Geometry: final body of the model. Coordinates: model frame, mm. Face numbers are marked on the shaded views. A direction names the side the tool comes from. Give positions to 0.01 mm unless a question says otherwise; leave off trailing zeros. Write each loop counter-clockwise with the first axis right and the second up, starting at its lowest first coordinate (ties: lowest second). Pieces come first, ordered by that corner, then holes. Notation, with made-up numbers: M 41.5,56 L 49.5,56 A25 cw 49.5,69 Z; hole C 39.25,-1.75 d2. An arc over 180 degrees is marked long. Use a Markdown table: item, result. Add a question column.
(1) Reachability of the marked faces 3 and 4 from +Z, -Z, +X, -X, +Y, -Y: full face, straight path, thin tool, end or side. Return the list, or none.
(2) Cut plane C-C (x = -583.5). Output: boundary loops of the cut face in (y, z).
(3) Draft query along Z for the marked faces 1 and 2. Return one class per face: released by +Z, released by -Z, zero draft, split by the parting line, or undercut.
(4) Cut plane D-D (z = -69.5). Output: boundary loops of the cut face in (x, y).
(5) Material intervals for L1, parallel to X at y = 31, z = -332.5; L2, parallel to Z at x = -277.5, y = 37.5; L3, parallel to Z at x = -638, y = 11.5, sorted ascending.
(6) Pin query (flat end, axial travel): pin 1 Ø12 at (x, z) = (-270, -61.5) entering from +Y; pin 2 Ø3.5 at (y, z) = (54, -441.5) entering from -X; pin 3 Ø2 at (y, z) = (14.5, -516.5) entering from +X; pin 4 Ø3.5 at (x, y) = (-68.5, 58.5) entering from +Z. Return the tip coordinate at first contact, or that it passes through.
(7) Cut plane B-B (x = -392). Output: boundary loops of the cut face in (y, z), plus the area to 3 significant figures.
(8) Cut plane A-A (z = -234). Output: boundary loops of the cut face in (x, y), plus the area to 3 significant figures.
Autodesk Inventor part; units mm, degrees
ref_plane "YZ Plane" through (0, 0, 0) normal (1, 0, 0) x (0, 1, 0)
ref_plane "XZ Plane" through (0, 0, 0) normal (0, 1, 0) x (-1, 0, 0)
ref_plane "XY Plane" through (0, 0, 0) normal (0, 0, 1) x (1, 0, 0)
sketch "Skizze1" plane through (0, 0, 0) normal (0, 1, 0) x (-1, 0, 0)
  line L0 (0, 0) -> (80, 0)
  line L1 (80, 0) -> (80, -650)
  line L2 (80, -650) -> (0, -650)
  line L3 (0, -650) -> (0, 0)
  line L4 (80, -570) -> (80, -650)
  line L5 (80, -650) -> (570, -650)
  line L6 (570, -650) -> (570, -570)
  line L7 (570, -570) -> (80, -570)
  line L8 (80, -570) -> (80, -650)
  line L9 (80, 0) -> (570, 0)
  line L10 (570, 0) -> (570, -80)
  line L11 (570, -80) -> (80, -80)
  line L12 (80, -80) -> (80, 0)
  line L13 (570, 0) -> (650, 0)
  line L14 (650, 0) -> (650, -650)
  line L15 (650, -650) -> (570, -650)
  line L16 (570, -650) -> (570, 0)
  dimension "d0" = 80
  dimension "d1" = 650
  dimension "d4" = 490
  dimension "d5" = 80
  dimension "d6" = 80
  dimension "d7" = 80
extrude "Extrusion1" add sketch "Skizze1" along normal blind 80 contours L0 L1 L2 L3 | L9 L10 L11 L1 | L13 L14 L15 L6 L16 L10 | L1 L7 L6 L5
sketch "Skizze2" plane through (0, 80, 0) normal (0, 1, 0) x (1, 0, 0)
  line L0 (0, 0) -> (0, 650)
  line L1 (0, 650) -> (-650, 650)
  line L2 (-650, 650) -> (-650, 0)
  line L3 (-650, 0) -> (0, 0)
  line L4 (-80, 80) -> (-570, 80)
  line L5 (-570, 80) -> (-570, 570)
  line L6 (-570, 570) -> (-80, 570)
  line L7 (-80, 570) -> (-80, 80)
  line L8 (-490, 305) -> (-490, 345)
  line L9 (-490, 345) -> (-650, 345)
  line L10 (-650, 345) -> (-650, 305)
  line L11 (-650, 305) -> (-490, 305)
  line L12 (-570, 80) -> (-570, 570)
  line L13 (-490, 305) -> (-650, 345) construction
  line L14 (-490, 345) -> (-650, 305) construction
  line L15 (-80, 80) -> (-570, 80)
  line L16 (-570, 80) -> (-270, 80)
  line L17 (-250, 160) -> (-290, 160)
  line L18 (-290, 160) -> (-290, 0)
  line L19 (-290, 0) -> (-250, 0)
  line L20 (-250, 0) -> (-250, 160)
  line L21 (-250, 160) -> (-290, 0) construction
  line L22 (-290, 160) -> (-250, 0) construction
  line L23 (-650, 325) -> (0, 325)
  line L24 (-250, 490) -> (-290, 490)
  line L25 (-290, 490) -> (-290, 650)
  line L26 (-250, 650) -> (-250, 490)
  line L27 (-290, 650) -> (-250, 650)
  point P0 (-570, 325)
  point P1 (-250, 570)
  point P2 (-290, 570)
  point P3 (-570, 345)
  point P4 (-570, 305)
  point P5 (-250, 80)
  point P6 (-290, 80)
  dimension "d10" = 40
  dimension "d11" = 300
  dimension "d12" = 40
extrude "Extrusion2" cut sketch "Skizze2" against normal blind 30 contours L3 L18 L4 L20 | L26 L6 L25 L1 | L23 L2 L9 L5 | L5 L11 L2 L23
sketch "Skizze3" plane through (0, 50, 0) normal (0, 1, 0) x (1, 0, 0)
  line L0 (-290, 80) -> (-250, 80)
  line L1 (-290, 0) -> (-290, 80)
  line L2 (-250, 0) -> (-290, 0)
  line L3 (-250, 80) -> (-250, 0)
  line L4 (-290, 650) -> (-250, 650)
  line L5 (-290, 570) -> (-290, 650)
  line L6 (-250, 570) -> (-290, 570)
  line L7 (-250, 650) -> (-250, 570)
  line L8 (-650, 345) -> (-570, 345)
  line L9 (-650, 305) -> (-650, 345)
  line L10 (-570, 305) -> (-650, 305)
  line L11 (-570, 345) -> (-570, 305)
  line L12 (-650, 305) -> (-625, 305)
  line L13 (-570, 305) -> (-650, 305)
  line L14 (-625, 305) -> (-625, 345)
  line L15 (-290, 650) -> (-290, 625)
  line L16 (-290, 570) -> (-290, 650)
  line L17 (-290, 625) -> (-250, 625)
  line L18 (-290, 0) -> (-290, 25)
  line L19 (-290, 25) -> (-250, 25)
  point P0 (0, 0)
  dimension "d15" = 25
  dimension "d16" = 25
  dimension "d17" = 25
extrude "Extrusion3" cut sketch "Skizze3" against normal blind 5 contours L0 L3 L19 L1 | L17 L7 L6 L5 | L8 L11 L10 L14
sketch "Skizze4" plane through (0, 0, -650) normal (0, 0, -1) x (-1, 0, 0)
  line L0 (290, 80) -> (290, 50)
  line L1 (290, 50) -> (250, 50)
  line L2 (250, 50) -> (250, 80)
  line L3 (0, 80) -> (250, 80)
  line L4 (0, 0) -> (0, 80)
  line L5 (0, 0) -> (650, 0)
  line L6 (650, 0) -> (650, 80)
  line L7 (290, 80) -> (650, 80)
  line L8 (250, 50) -> (250, 45)
  line L9 (250, 50) -> (0, 50)
  line L10 (0, 0) -> (0, 80)
  line L11 (290, 50) -> (250, 50)
  line L12 (250, 50) -> (250, 62)
  line L13 (250, 62) -> (0, 62)
  line L14 (290, 50) -> (650, 50)
  line L15 (290, 62) -> (650, 62)
  dimension "d20" = 12
extrude "Extrusion4" cut sketch "Skizze4" against normal blind 12 contours L15 L6 L14 L0 | L9 L4 L13 L2
sketch "Skizze5" plane through (-650, 0, -650) normal (-1, 0, 0) x (0, 0, 1)
  line L0 (12, 50) -> (0, 50)
  line L1 (0, 0) -> (0, 50)
  line L2 (0, 0) -> (650, 0)
  line L3 (650, 0) -> (650, 80)
  line L4 (345, 80) -> (650, 80)
  line L5 (345, 80) -> (345, 50)
  line L6 (345, 50) -> (305, 50)
  line L7 (305, 50) -> (305, 80)
  line L8 (0, 80) -> (305, 80)
  line L9 (0, 62) -> (0, 80)
  line L10 (0, 62) -> (12, 62)
  line L11 (12, 62) -> (12, 50)
  line L12 (12, 50) -> (650, 50)
  line L13 (12, 62) -> (650, 62)
  point P0 (345, 62)
  point P1 (305, 62)
extrude "Extrusion5" cut sketch "Skizze5" against normal blind 12 contours L11 L13 L7 L12 | L5 L13 L3 L12
sketch "Skizze6" plane through (-650, 0, 0) normal (0, 0, 1) x (1, 0, 0)
  line L0 (12, 50) -> (12, 62)
  line L1 (12, 50) -> (650, 50)
  line L2 (360, 62) -> (12, 62)
  line L3 (650, 62) -> (400, 62)
  line L4 (12, 50) -> (0, 50)
  line L5 (0, 0) -> (0, 50)
  line L6 (0, 0) -> (650, 0)
  line L7 (650, 0) -> (650, 80)
  line L8 (400, 80) -> (650, 80)
  line L9 (400, 80) -> (400, 50)
  line L10 (400, 50) -> (360, 50)
  line L11 (360, 50) -> (360, 80)
  line L12 (0, 80) -> (360, 80)
  line L13 (0, 62) -> (0, 80)
  line L14 (0, 62) -> (12, 62)
  line L15 (12, 62) -> (12, 50)
extrude "Extrusion6" cut sketch "Skizze6" against normal blind 12 contours L0 L2 L11 L1 | L9 L3 L7 L1
sketch "Skizze7" plane through (0, 0, -650) normal (0, 0, -1) x (-1, 0, 0)
  line L0 (650, 50) -> (0, 50)
  line L1 (0, 0) -> (0, 50)
  line L2 (0, 0) -> (650, 0)
  line L3 (650, 0) -> (650, 50)
  line L4 (0, 50) -> (0, 62)
  line L5 (250, 50) -> (0, 50)
  line L6 (250, 62) -> (250, 50)
  line L7 (0, 62) -> (250, 62)
  line L8 (0, 62) -> (250, 62)
  line L9 (250, 62) -> (250, 80)
  line L10 (0, 80) -> (250, 80)
  line L11 (0, 62) -> (0, 80)
  line L12 (290, 62) -> (650, 62)
  line L13 (650, 62) -> (650, 80)
  line L14 (290, 80) -> (650, 80)
  line L15 (290, 80) -> (290, 62)
  line L16 (638, 50) -> (638, 62)
  line L17 (290, 62) -> (638, 62)
  line L18 (290, 50) -> (290, 62)
  line L19 (638, 50) -> (290, 50)
  line L20 (250, 50) -> (200, 50)
  line L21 (290, 50) -> (340, 50)
  line L22 (250, 50) -> (290, 50)
  ellipse E0 centre (270, 50) end of major axis (200, 50) minor radius 17.9197
  line L23 (200, 50) -> (188, 50)
  line L24 (250, 62) -> (0, 62)
  line L25 (218.0128, 62) -> (213.5364, 73.1338)
  ellipse E1 centre (270, 50) end of major axis (188, 50) minor radius 28.5733
  point P0 (352, 50)
  dimension "d27" = 50
  dimension "d28" = 50
  dimension "d29" = 12
  dimension "d30" = 12
extrude "Extrusion7" cut sketch "Skizze7" against normal blind 12 contours E1 L0 E0
sketch "Skizze8" plane through (0, 50, 0) normal (0, 1, 0) x (1, 0, 0)
  line L0 (-352, 638) -> (-352, 650)
  line L1 (-650, 650) -> (-352, 650)
  line L2 (-650, 0) -> (-650, 650)
  line L3 (0, 0) -> (-650, 0)
  line L4 (0, 12) -> (0, 0)
  line L5 (0, 12) -> (-250, 12)
  line L6 (-250, 25) -> (-250, 12)
  line L7 (-250, 25) -> (-290, 25)
  line L8 (-290, 12) -> (-290, 25)
  line L9 (-290, 12) -> (-638, 12)
  line L10 (-638, 12) -> (-638, 305)
  line L11 (-625, 305) -> (-638, 305)
  line L12 (-625, 305) -> (-625, 345)
  line L13 (-638, 345) -> (-625, 345)
  line L14 (-638, 345) -> (-638, 638)
  line L15 (-638, 638) -> (-352, 638)
  line L16 (-290, 25) -> (-290, 80)
  line L17 (-250, 25) -> (-290, 25)
  line L18 (-250, 80) -> (-250, 25)
  line L19 (-290, 80) -> (-250, 80)
  line L20 (-290, 0) -> (-290, 12)
  line L21 (-290, 12) -> (-290, 0)
  line L22 (0, 12) -> (-250, 12)
  line L23 (-250, 80) -> (-250, 0)
  line L24 (-250, 12) -> (-250, 0)
  line L25 (-250, 12) -> (-262.5, 12)
  line L26 (-262.5, 12) -> (-277.5, 12)
  circle A0 centre (-277.5, 12) radius 3
  circle A1 centre (-262.5, 12) radius 3
  line L27 (-638, 305) -> (-638, 317.5)
  line L28 (-638, 317.5) -> (-638, 332.5)
  circle A2 centre (-638, 317.5) radius 3
  circle A3 centre (-638, 332.5) radius 3
  line L29 (-340, 650) -> (-340, 638)
  line L30 (-340, 638) -> (-290, 638)
  line L31 (-290, 625) -> (-290, 638)
  line L32 (-290, 625) -> (-250, 625)
  line L33 (-250, 638) -> (-250, 625)
  line L34 (-250, 638) -> (-200, 638)
  line L35 (-200, 638) -> (-200, 650)
  line L36 (-340, 650) -> (-200, 650)
  line L37 (-290, 638) -> (-290, 625.5)
  line L38 (-290, 570) -> (-290, 650)
  line L39 (-290, 638) -> (-277.5, 638)
  line L40 (-277.5, 638) -> (-262.5, 638)
  circle A4 centre (-277.5, 638) radius 3
  circle A5 centre (-262.5, 638) radius 3
  dimension "d35" = 12.5
  dimension "d36" = 15
  dimension "d37" = 6
  dimension "d38" = 6
  dimension "d39" = 12.5
  dimension "d40" = 15
  dimension "d41" = 6
  dimension "d42" = 6
  dimension "d43" = 12.5
  dimension "d44" = 12.5
  dimension "d45" = 15
  dimension "d46" = 6
  dimension "d47" = 6
extrude "Extrusion8" cut sketch "Skizze8" against normal blind 100 contours A3 | A2 L28 L27 | L27 L28 A2 | A0 | A1 L26 L25 | L25 L26 A1 | A5 | A4 L40 L39 | L39 L40 A4
properties part number "Rahmen_Unten" material "Holz (Birke)"
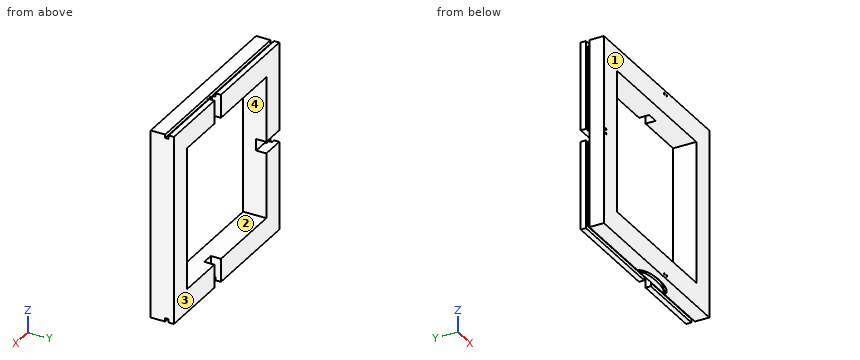
Answer list:
| question | item | result |
|---|---|---|
| 1 | face 3 | +Z, -Z, +X, -X, +Y |
| 1 | face 4 | +Y, -Y |
| 2 | outline | M 0,-650 L 50,-650 L 50,-638 L 62,-638 L 62,-650 L 80,-650 L 80,-345 L 45,-345 L 45,-305 L 80,-305 L 80,0 L 62,0 L 62,-12 L 50,-12 L 50,0 L 0,0 Z |
| 3 | face 1 | zero draft |
| 3 | face 2 | undercut |
| 4 | outline | M -650,0 L 0,0 L 0,80 L -250,80 L -250,45 L -290,45 L -290,80 L -650,80 L -650,62 L -638,62 L -638,50 L -650,50 Z |
| 5 | L1 | -650 to -641, -635 to -570, -80 to 0 |
| 5 | L2 | -650 to -641, -635 to -570, -80 to -15, -9 to 0 |
| 5 | L3 | -650 to -335.5, -329.5 to -320.5, -314.5 to 0 |
| 6 | pin 1 | y = 45 |
| 6 | pin 2 | x = -638 |
| 6 | pin 3 | x = 0 |
| 6 | pin 4 | z = -12 |
| 7 | outline | M 0,-650 L 50,-650 L 50,-638 L 62,-638 L 62,-650 L 80,-650 L 80,-570 L 0,-570 Z; M 0,-80 L 80,-80 L 80,0 L 62,0 L 62,-12 L 50,-12 L 50,0 L 0,0 Z |
| 7 | area | 12,500 mm² |
| 8 | outline | M -650,0 L -570,0 L -570,80 L -650,80 L -650,62 L -638,62 L -638,50 L -650,50 Z; M -80,0 L 0,0 L 0,80 L -80,80 Z |
| 8 | area | 12,700 mm² |
